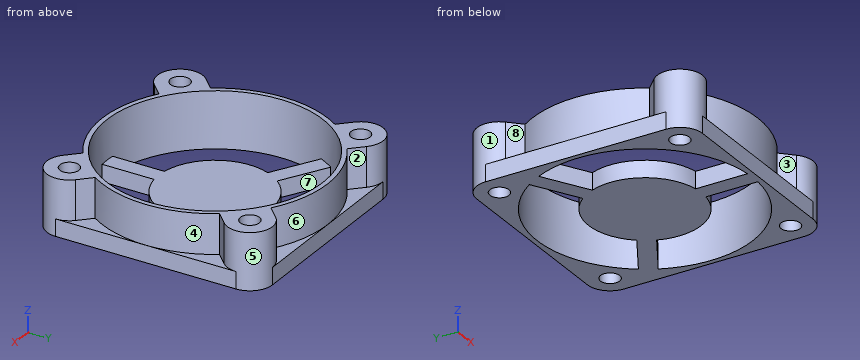
from build123d import *

# Parameters (mm, degrees)
SKETCH_BODY_R                       = 19.15
BODY_DEPTH                          = 10
SKETCH_CUT_BODY_W                   = 7
SKETCH_CUT_BODY_H                   = 6.627416998
REINFORCMENT_STRIP_DEPTH            = 10
CIRPATTERN_REINFORCMENT_STRIP_COUNT = 4
SKETCH_FIXING_HOLE_R                = 1.7
FIXING_HOLE_DEPTH                   = 31
CIRPATTERN_FIXING_HOLE_COUNT        = 4
BONE_DEPTH                          = 3
CIRPATTERN_BONE_COUNT               = 3
SKETCH_FIXING_PLATE_FAN_R           = 10
FIXING_PLATE_FAN_DEPTH              = 3


with BuildPart() as part:
    # Sketch-Body → Body (new body)
    with BuildSketch(Plane.XY):
        with BuildLine():
            Line((-16, -20), (16, -20))
            ThreePointArc((16, -20), (18.828427125, -18.828427125), (20, -16))
            Line((20, -16), (20, 16))
            ThreePointArc((20, 16), (18.828427125, 18.828427125), (16, 20))
            Line((16, 20), (-16, 20))
            ThreePointArc((-16, 20), (-18.828427125, 18.828427125), (-20, 16))
            Line((-20, 16), (-20, -16))
            ThreePointArc((-20, -16), (-18.828427125, -18.828427125), (-16, -20))
        make_face()
        with Locations(Location((0, 0, 0), (0, 0, 180))):
            Circle(SKETCH_BODY_R, mode=Mode.SUBTRACT)
    extrude(amount=BODY_DEPTH)

    # Sketch-Cut-Body → Cut-Body (revolve, cut)
    with BuildSketch(Plane(origin=(0, 0, 0), x_dir=(0, 0, -1), z_dir=(1, 0, 0)), mode=Mode.PRIVATE) as cut_body_sk:
        with Locations((-6.5, 23.313708499)):
            Rectangle(SKETCH_CUT_BODY_W, SKETCH_CUT_BODY_H)
    revolve(cut_body_sk.sketch.rotate(Axis((0, 0, 10), (0, 0, -1)), 90), axis=Axis((0, 0, 10), (0, 0, -1)), mode=Mode.SUBTRACT)

    # Sketch-Reinforcment-Strip → Reinforcment-Strip (add)
    with BuildSketch(Plane.XY):
        with BuildLine():
            Line((16.684833585, 11.027979336), (18.828427125, 13.171572875))
            ThreePointArc((18.828427125, 13.171572875), (18.828427125, 18.828427125), (13.171572875, 18.828427125))
            Line((13.171572875, 18.828427125), (11.027979336, 16.684833585))
            ThreePointArc((11.027979336, 16.684833585), (14.142135624, 14.142135624), (16.684833585, 11.027979336))
        make_face()
    reinforcment_strip = extrude(amount=REINFORCMENT_STRIP_DEPTH)

    # CirPattern-Reinforcment-Strip: Reinforcment-Strip ×4 about axis
    cirpattern_reinforcment_strip_axis = Axis((0, 0, 0), (0, 0, 1))
    for i in range(1, CIRPATTERN_REINFORCMENT_STRIP_COUNT):
        add(reinforcment_strip.rotate(cirpattern_reinforcment_strip_axis, i * 360 / CIRPATTERN_REINFORCMENT_STRIP_COUNT))

    # Sketch-Fixing-Hole → Fixing-Hole (cut, through all)
    with BuildSketch(Plane.XY):
        with Locations((16, 16)):
            Circle(SKETCH_FIXING_HOLE_R)
    fixing_hole = extrude(amount=FIXING_HOLE_DEPTH, mode=Mode.SUBTRACT)

    # CirPattern-Fixing-Hole: Fixing-Hole ×4 about axis
    cirpattern_fixing_hole_axis = Axis((0, 0, 0), (0, 0, 1))
    for i in range(1, CIRPATTERN_FIXING_HOLE_COUNT):
        add(fixing_hole.rotate(cirpattern_fixing_hole_axis, i * 360 / CIRPATTERN_FIXING_HOLE_COUNT), mode=Mode.SUBTRACT)

    # Sketch-Bone → Bone (add)
    with BuildSketch(Plane.XY):
        with BuildLine():
            Line((1.5, -9.886859967), (1.5, -19.091162877))
            ThreePointArc((1.5, -19.091162877), (0, -19.15), (-1.5, -19.091162877))
            Line((-1.5, -19.091162877), (-1.5, -9.886859967))
            ThreePointArc((-1.5, -9.886859967), (0, -10), (1.5, -9.886859967))
        make_face()
    bone = extrude(amount=BONE_DEPTH)

    # CirPattern-Bone: Bone ×3 about axis
    cirpattern_bone_axis = Axis((0, 0, 0), (0, 0, 1))
    for i in range(1, CIRPATTERN_BONE_COUNT):
        add(bone.rotate(cirpattern_bone_axis, i * 360 / CIRPATTERN_BONE_COUNT))

    # Sketch-Fixing-Plate-Fan → Fixing-Plate-Fan (add)
    with BuildSketch(Plane.XY):
        Circle(SKETCH_FIXING_PLATE_FAN_R)
    extrude(amount=FIXING_PLATE_FAN_DEPTH)


solid = part.part
The listing builds one solid part. Answer for the finished solid, in the listing's coordinates (mm). Face numbers are marked on the shaded views. A direction names the side the tool comes from. Coordinates: 2 decimals unless noted, no trailing zeros. Loops run counter-clockwise (first coordinate to the right, second up) from the corner with the lowest first, then second, coordinate; pieces in that order, holes last. Notation, with made-up numbers: M 84,34 L 136,34 A24 ccw 136,67 Z; hole C 48,-24.75 d6. An arc over 180 degrees is marked long. Answer in a Markdown table with one row per item.
1) Which of the six approach directions +Z, -Z, +X, -X, +Y, -Y give full straight-line access (tool end or side, diameter ignored) to the marked faces 4, 5, 6, 7 and 8?
Answers below:
| item | result |
|---|---|
| face 4 | +Z, +X |
| face 5 | +Z |
| face 6 | +Z, +Y |
| face 7 | +Z, -Z |
| face 8 | +Z, -X |
2) Find section A-A (z = 2.5). Determine the outline of the cut face in (x, y).
Answers below:
| item | result |
|---|---|
| outline | M -20,-16 A4 ccw -16,-20 L 16,-20 A4 ccw 20,-16 L 20,16 A4 ccw 16,20 L -16,20 A4 ccw -20,16 Z; hole C -16,-16 d3.4; hole C -16,16 d3.4; hole M -17.28,8.25 A19.15 ccw -1.5,-19.09 L -1.5,-9.89 A10 cw -9.31,3.64 Z; hole M -15.78,10.84 L -7.81,6.24 A10 cw 7.81,6.24 L 15.78,10.84 A19.15 ccw Z; hole M 1.5,-19.09 A19.15 ccw 17.28,8.25 L 9.31,3.64 A10 cw 1.5,-9.89 Z; hole C 16,-16 d3.4; hole C 16,16 d3.4 |
3) Find section C-C (z = 7.25). Determine the outline of the cut face in (x, y), then the cut area to 3 significant figures.
Answers below:
| item | result |
|---|---|
| outline | M -18.83,-13.17 A4 ccw -13.17,-18.83 L -11.03,-16.68 A20 ccw 11.03,-16.68 L 13.17,-18.83 A4 ccw 18.83,-13.17 L 16.68,-11.03 A20 ccw 16.68,11.03 L 18.83,13.17 A4 ccw 13.17,18.83 L 11.03,16.68 A20 ccw -11.03,16.68 L -13.17,18.83 A4 ccw -18.83,13.17 L -16.68,11.03 A20 ccw -16.68,-11.03 Z; hole C 0,0 d38.3; hole C -16,-16 d3.4; hole C -16,16 d3.4; hole C 16,-16 d3.4; hole C 16,16 d3.4 |
| area | 257 mm^2 |
4) Determine the mould class of the marked faces 1, 2 and 3 for opening direction Y: released by +Y, released by -Y, zero draft, split by the parting line, or undercut.
Answers below:
| item | result |
|---|---|
| face 1 | undercut |
| face 2 | released by +Y |
| face 3 | released by -Y |
5) Find section B-B (y = -10.5). Determine the outline of the cut face in (x, z).
Answers below:
| item | result |
|---|---|
| outline | M -20,0 L -16.01,0 L -16.01,10 L -17.02,10 L -17.02,3 L -20,3 Z; M -1.5,0 L 1.5,0 L 1.5,3 L -1.5,3 Z; M 16.01,0 L 20,0 L 20,3 L 17.02,3 L 17.02,10 L 16.01,10 Z |
6) Find the intervals of material crossed by probe 1 along Y at (x, z) = (13, 2.5); probe 2 along Y at (x, z) = (0, 6); probe 3 along Y at (x, z) = (14.5, 6), in increasing order.
Answers below:
| item | result |
|---|---|
| probe 1 | -20 to -14.06, 5.77 to 9.24, 14.06 to 20 |
| probe 2 | -20 to -19.15, 19.15 to 20 |
| probe 3 | -19.71 to -16.8, -15.2 to -12.51, 12.51 to 15.2, 16.8 to 19.71 |
7) Given pin 1 (15 mm diameter, centred on x = -1, y = -1.5, fed in from +Z), flat-ended and moving along its own axis, determine where the tip first touches the part or whether it passes through.
Answers below:
| item | result |
|---|---|
| pin 1 | z = 3 |
8) Find section D-D (x = 12.5). Determine the outline of the cut face in (y, z), then the cut area to 3 significant figures.
Answers below:
| item | result |
|---|---|
| outline | M -20,0 L -14.51,0 L -14.51,10 L -18.16,10 L -18.16,3 L -20,3 Z; M 5.48,0 L 8.95,0 L 8.95,3 L 5.48,3 Z; M 14.51,0 L 20,0 L 20,3 L 18.16,3 L 18.16,10 L 14.51,10 Z |
| area | 94.4 mm^2 |
